Can you work these out from the model? Positions are in its coordinate system, mm. A direction names the side the tool comes from. Give positions to 0.01 mm unless a question says otherwise; leave off trailing zeros. Write each loop counter-clockwise with the first axis right and the second up, starting at its lowest first coordinate (ties: lowest second). Pieces come first, ordered by that corner, then holes. Notation, with made-up numbers: M 7.25,79.25 L 56.25,79.25 A28 cw 56.25,112.25 Z; hole C 21.25,-20.5 d5. An arc over 180 degrees is marked long. Answer as CSV lines item,"result". Start each with the question number.
```python
from build123d import *

# Parameters (mm, degrees)
SKETCH1_W           = 25.4
SKETCH1_H           = 50.8
SKETCH1_W_2         = 20.32
SKETCH1_H_2         = 45.72
BOSS_EXTRUDE1_DEPTH = 203.2
SKETCH2_R           = 0.5
CUT_EXTRUDE1_DEPTH  = 26.4


with BuildPart() as part:
    # Sketch1 → Boss-Extrude1 (new body)
    with BuildSketch(Plane.XY):
        with Locations((16.665400844, -8.681012658)):
            Rectangle(SKETCH1_W, SKETCH1_H)
        with Locations((16.665400844, -8.681012658)):
            Rectangle(SKETCH1_W_2, SKETCH1_H_2, mode=Mode.SUBTRACT)
    extrude(amount=BOSS_EXTRUDE1_DEPTH)

    # Sketch2 → Cut-Extrude1 (cut, through all)
    with BuildSketch(Plane(origin=(29.365400844, 0, 0), x_dir=(0, 0, -1), z_dir=(1, 0, 0))):
        with Locations((-190.5, 4.018987342)):
            Circle(SKETCH2_R)
        with Locations((-177.8, 4.018987342)):
            Circle(SKETCH2_R)
        with Locations((-165.1, 4.018987342)):
            Circle(SKETCH2_R)
        with Locations((-152.4, 4.018987342)):
            Circle(SKETCH2_R)
        with Locations((-139.7, 4.018987342)):
            Circle(SKETCH2_R)
        with Locations((-127, 4.018987342)):
            Circle(SKETCH2_R)
        with Locations((-114.3, 4.018987342)):
            Circle(SKETCH2_R)
        with Locations((-101.6, 4.018987342)):
            Circle(SKETCH2_R)
        with Locations((-88.9, 4.018987342)):
            Circle(SKETCH2_R)
        with Locations((-76.2, 4.018987342)):
            Circle(SKETCH2_R)
        with Locations((-63.5, 4.018987342)):
            Circle(SKETCH2_R)
        with Locations((-50.8, 4.018987342)):
            Circle(SKETCH2_R)
        with Locations((-38.1, 4.018987342)):
            Circle(SKETCH2_R)
        with Locations((-25.4, 4.018987342)):
            Circle(SKETCH2_R)
        with Locations((-12.7, 4.018987342)):
            Circle(SKETCH2_R)
        with Locations((-177.8, -8.681012658)):
            Circle(SKETCH2_R)
        with Locations((-165.1, -8.681012658)):
            Circle(SKETCH2_R)
        with Locations((-152.4, -8.681012658)):
            Circle(SKETCH2_R)
        with Locations((-139.7, -8.681012658)):
            Circle(SKETCH2_R)
        with Locations((-127, -8.681012658)):
            Circle(SKETCH2_R)
        with Locations((-114.3, -8.681012658)):
            Circle(SKETCH2_R)
        with Locations((-101.6, -8.681012658)):
            Circle(SKETCH2_R)
        with Locations((-88.9, -8.681012658)):
            Circle(SKETCH2_R)
        with Locations((-76.2, -8.681012658)):
            Circle(SKETCH2_R)
        with Locations((-63.5, -8.681012658)):
            Circle(SKETCH2_R)
        with Locations((-50.8, -8.681012658)):
            Circle(SKETCH2_R)
        with Locations((-38.1, -8.681012658)):
            Circle(SKETCH2_R)
        with Locations((-25.4, -8.681012658)):
            Circle(SKETCH2_R)
        with Locations((-12.7, -8.681012658)):
            Circle(SKETCH2_R)
        with Locations((-177.8, -21.381012658)):
            Circle(SKETCH2_R)
        with Locations((-165.1, -21.381012658)):
            Circle(SKETCH2_R)
        with Locations((-152.4, -21.381012658)):
            Circle(SKETCH2_R)
        with Locations((-139.7, -21.381012658)):
            Circle(SKETCH2_R)
        with Locations((-127, -21.381012658)):
            Circle(SKETCH2_R)
        with Locations((-114.3, -21.381012658)):
            Circle(SKETCH2_R)
        with Locations((-101.6, -21.381012658)):
            Circle(SKETCH2_R)
        with Locations((-88.9, -21.381012658)):
            Circle(SKETCH2_R)
        with Locations((-76.2, -21.381012658)):
            Circle(SKETCH2_R)
        with Locations((-63.5, -21.381012658)):
            Circle(SKETCH2_R)
        with Locations((-50.8, -21.381012658)):
            Circle(SKETCH2_R)
        with Locations((-38.1, -21.381012658)):
            Circle(SKETCH2_R)
        with Locations((-25.4, -21.381012658)):
            Circle(SKETCH2_R)
        with Locations((-12.7, -21.381012658)):
            Circle(SKETCH2_R)
        with Locations((-190.5, -8.681012658)):
            Circle(SKETCH2_R)
        with Locations((-190.5, -21.381012658)):
            Circle(SKETCH2_R)
    extrude(amount=-CUT_EXTRUDE1_DEPTH, mode=Mode.SUBTRACT)


solid = part.part
```
1) I'm going to push a flat-ended pin straight in: P1, Ø1.5, axis at x = 9, y = -20.5, coming from the -Z side. Where does the tip first touch, or does it pass through?
2) Thinking about a two-plate mould opening in X: for faces 1 (the flat face through (16, -34.081, 100)), 2 (the flat face through (17, 14.179, 100)), 3 (the flat face through (29.365, -9, 100)), 4 (the flat face through (3.965, -9, 100)), which applies, released by +X, released by -X, zero draft, split by the parting line, or undercut?
3) I need wall thicknesses on L1, parallel to Y at x = 28.6, z = 165.1; L2, parallel to Y at x = 16, z = 133; L3, parallel to X at y = 1, z = 180. Which ranges of each line are inside material? Lowest first, please. Write a range as from..to.
4) I want a section at C-C, the plane z = 19. Please give me the cut outline in (x, y).
5) I want a section at B-B, the plane y = -13. Please give me the cut outline in (x, z).
6) On a 3-axis mill with a long thin cutter (end or side, diameter ignored), from which of +Z, -Z, +X, -X, +Y, -Y can I reach the whole of each face in a straight line? I mean faces 5 (the flat face through (26.825, -9, 100)), 6 (the flat face through (6, -7, 0)). Say none if no direction works.
7) I want a section at A-A, the plane x = 18. Please give me the cut outline in (y, z), then the cut area to 3 significant figures.
Values found:
1,P1,"passes through"
2,face 1,"zero draft"
2,face 2,"undercut"
2,face 3,"released by +X"
2,face 4,"released by -X"
3,L1,"y = -34.08..-21.88, -20.88..-9.18, -8.18..3.52, 4.52..16.72"
3,L2,"y = -34.08..-31.54, 14.18..16.72"
3,L3,"x = 3.97..6.51, 26.83..29.37"
4,outline,"M 3.97,-34.08 L 29.37,-34.08 L 29.37,16.72 L 3.97,16.72 Z; hole M 6.51,-31.54 L 26.83,-31.54 L 26.83,14.18 L 6.51,14.18 Z"
5,outline,"M 3.97,0 L 6.51,0 L 6.51,203.2 L 3.97,203.2 Z; M 26.83,0 L 29.37,0 L 29.37,203.2 L 26.83,203.2 Z"
6,face 5,"+Z, -Z"
6,face 6,"-Z, +X, -X, +Y, -Y"
7,outline,"M -34.08,0 L -31.54,0 L -31.54,203.2 L -34.08,203.2 Z; M 14.18,0 L 16.72,0 L 16.72,203.2 L 14.18,203.2 Z"
7,area,"1,030 mm²"
